```python
from build123d import *

# Parameters (mm, degrees)
F0_W     = 38.1
F0_H     = 38.1
F1_DEPTH = 38.1
F2_W     = 33.02
F2_H     = 33.02
F3_DEPTH = 35.56
F4_R     = 2.54
F5_R     = 12.065
F6_DEPTH = 38.101
F7_R     = 1.26999


# Not quite as in the source:
# - a fillet or chamfer is up to 0.001 mm smaller than in the source, because OpenCascade refuses the exact size


with BuildPart() as f1:
    # F0 (on Top) → F1 (new body)
    with BuildSketch(Plane.XY):
        with Locations((19.05, -19.05)):
            Rectangle(F0_W, F0_H)
    extrude(amount=F1_DEPTH)

    # F2 (on face) → F3 (cut)
    with BuildSketch(Plane(origin=(0, 0, 0), x_dir=(1, 0, 0), z_dir=(0, 0, -1))):
        with Locations((19.05, 19.05)):
            Rectangle(F2_W, F2_H)
    extrude(amount=-F3_DEPTH, mode=Mode.SUBTRACT)

    # F4
    f4_edges = [f1.edges().sort_by_distance(p)[0] for p in [
        (19.05, -35.56, 35.56),
        (2.54, -19.05, 35.56),
        (35.56, -19.05, 35.56),
        (19.05, -2.54, 35.56),
    ]]
    fillet(f4_edges, radius=F4_R)

    # F5 (on face) → F6 (cut, through all)
    with BuildSketch(Plane(origin=(0, 0, 0), x_dir=(-1, 0, 0), z_dir=(0, 1, 0))):
        with Locations((-19.05, 19.05)):
            Circle(F5_R)
    extrude(amount=-F6_DEPTH, mode=Mode.SUBTRACT)

    # F7 (radius 1.27 in the source; OpenCascade refuses exactly that, so slightly less here)
    f7_edges = [f1.edges().sort_by_distance(p)[0] for p in [
        (31.115, 0, 19.05),
        (31.115, -2.54, 19.05),
        (31.115, -35.56, 19.05),
        (31.115, -38.1, 19.05),
    ]]
    fillet(f7_edges, radius=F7_R)


solid = f1.part
```
Geometry check sheet. Reference: the model listing, model coordinates, mm. A direction names the side the tool comes from. Give positions to 0.01 mm unless a question says otherwise; leave off trailing zeros. Write each loop counter-clockwise with the first axis right and the second up, starting at its lowest first coordinate (ties: lowest second). Pieces come first, ordered by that corner, then holes.
1) Material ranges on L1, parallel to X at y = -4.5, z = 11.5; L2, parallel to Y at x = 27.5, z = 5.5; L3, parallel to Z at x = 19.05, y = -1.25, recorded low to high.
2) Release check for a two-part mould opening along Y. For faces 1 (the flat face through (0, -19, 19)), 2 (the flat face through (6, -38.1, 15)), 3 (the flat face through (2.54, -19, 16)) record: pulls with the +Y half, pulls with the -Y half, needs draft (parallel to the pull), parting line crosses it, or undercut.
3) Access from +Z, -Z, +X, -X, +Y, -Y to the whole of each face (thin tool, end or side, straight path). Record for faces 4 (the flat face through (19, -19, 38.1)), 5 (the flat face through (19, -19, 35.56)).
4) Section check B-B, the plane y = -12. Record the boundary of the cut face in (x, z).
5) Section check A-A, the plane x = 19.05. State how many separate pieces and enclosed holes the cut face has, and give its area (3 significant figures).
6) Gauge pin test, flat ends, axial feed: pin 1 (5 mm diameter, centred on x = 14, z = 13.5, fed in from +Y); pin 2 (6 mm diameter, centred on x = 10, z = 16.5, fed in from +Y); pin 3 (8.5 mm diameter, centred on x = 17.5, y = -21.5, fed in from -Z). Record the tip position at first contact, or that the pin passes through.
Computed:
1. L1: x = 0 to 2.54, 35.56 to 38.1
1. L2: y = -38.1 to -35.56, -2.54 to 0
1. L3: z = 0 to 6.98, 31.12 to 38.1
2. face 1: needs draft
2. face 2: pulls with the -Y half
2. face 3: undercut
3. face 4: +Z, +X, -X, +Y, -Y
3. face 5: -Z
4. outline: (0, 0) - (2.54, 0) - (2.54, 33.02) arc R2.54 cw to (5.08, 35.56) - (33.02, 35.56) arc R2.54 cw to (35.56, 33.02) - (35.56, 0) - (38.1, 0) - (38.1, 38.1) - (0, 38.1) - close
5. separate pieces: 3
5. enclosed holes: 0
5. area: 155 mm2
6. pin 1: passes through
6. pin 2: stops at y = -0.41
6. pin 3: stops at z = 35.56
